Autodesk Inventor part; units mm, degrees
ref_plane "YZ Plane" through (0, 0, 0) normal (1, 0, 0) x (0, 1, 0)
ref_plane "XZ Plane" through (0, 0, 0) normal (0, 1, 0) x (-1, 0, 0)
ref_plane "XY Plane" through (0, 0, 0) normal (0, 0, 1) x (1, 0, 0)
sketch "Sketch1" plane through (0, 0, 0) normal (1, 0, 0) x (0, 1, 0)
  line L0 (-6, -12.5) -> (-6, -12.9)
  arc A0 (-6, -12.9) -> (-5.6, -13.3) centre (-5.6, -12.9) ccw
  line L1 (-5.6, -13.3) -> (-4.9, -13.3)
  arc A1 (-4.9, -13.3) -> (-4.7, -13.1) centre (-4.9, -13.1) ccw
  line L2 (-4.7, -13.1) -> (-4.7, -12.85)
  arc A2 (-4.5, -12.65) -> (-4.7, -12.85) centre (-4.5, -12.85) ccw
  line L3 (-4.5, -12.65) -> (-1.8, -12.65)
  arc A3 (-1.4, -13.05) -> (-1.8, -12.65) centre (-1.8, -13.05) ccw
  line L4 (-1.4, -13.05) -> (-1.4, -18.75)
  line L5 (-1.8, -19.15) -> (-4.5, -19.15)
  arc A4 (-1.8, -19.15) -> (-1.4, -18.75) centre (-1.8, -18.75) ccw
  arc A5 (-4.7, -18.95) -> (-4.5, -19.15) centre (-4.5, -18.95) ccw
  line L6 (-4.7, -18.95) -> (-4.7, -18.7)
  arc A6 (-4.7, -18.7) -> (-4.9, -18.5) centre (-4.9, -18.7) ccw
  line L7 (-4.9, -18.5) -> (-5.6, -18.5)
  arc A7 (-5.6, -18.5) -> (-6, -18.9) centre (-5.6, -18.9) ccw
  line L8 (-6, -18.9) -> (-6, -19.5)
  line L9 (-6.5, -6.5) -> (-6.5, -12.5)
  line L10 (-6.5, -12.5) -> (-2.5, -12.5)
  line L11 (-1.05, -19.5) -> (-6.5, -19.5)
  line L12 (-6.5, -19.5) -> (-6.5, -26)
  line L13 (-6.5, -26) -> (-1.05, -26)
  line L14 (-6, -26) -> (-6, -26.6)
  arc A8 (-6, -26.6) -> (-5.6, -27) centre (-5.6, -26.6) ccw
  line L15 (-5.6, -27) -> (-4.9, -27)
  arc A9 (-4.9, -27) -> (-4.7, -26.8) centre (-4.9, -26.8) ccw
  arc A10 (-4.5, -26.35) -> (-4.7, -26.55) centre (-4.5, -26.55) ccw
  line L16 (-4.7, -26.8) -> (-4.7, -26.55)
  line L17 (-4.5, -26.35) -> (-1.8, -26.35)
  arc A11 (-1.4, -26.75) -> (-1.8, -26.35) centre (-1.8, -26.75) ccw
  line L18 (-1.4, -26.75) -> (-1.4, -32.45)
  arc A12 (-1.8, -32.85) -> (-1.4, -32.45) centre (-1.8, -32.45) ccw
  line L19 (-1.8, -32.85) -> (-4.5, -32.85)
  arc A13 (-4.7, -32.65) -> (-4.5, -32.85) centre (-4.5, -32.65) ccw
  line L20 (-4.7, -32.65) -> (-4.7, -32.4)
  arc A14 (-4.7, -32.4) -> (-4.9, -32.2) centre (-4.9, -32.4) ccw
  line L21 (-4.9, -32.2) -> (-5.6, -32.2)
  arc A15 (-5.6, -32.2) -> (-6, -32.6) centre (-5.6, -32.6) ccw
  line L22 (-6, -32.6) -> (-6, -33)
  line L23 (-2.5, -33) -> (-6.5, -33)
  line L24 (-6.5, -33) -> (-6.5, -39)
  line L25 (32.5, 0) -> (0, 0)
  circle A16 centre (0, -6.5) radius 4.75
  circle A17 centre (32.5, -6.5) radius 4.75
  circle A18 centre (0, -39) radius 4.75
  circle A19 centre (32.5, -39) radius 4.75
  line L26 (39, -26) -> (39, -19.5)
  line L27 (39, -12.5) -> (39, -6.5)
  line L28 (39, -39) -> (39, -33)
  line L29 (26.5, -45.5) -> (32.5, -45.5)
  line L30 (0, -45.5) -> (6, -45.5)
  line L31 (13, -45.5) -> (19.5, -45.5)
  circle A20 centre (16.25, -22.75) radius 15
  circle A21 centre (16.2588, 5.0016) radius 2.5
  circle A22 centre (16.25, -50.5) radius 2.5
  circle A23 centre (16.25, -22.75) radius 5
  circle A24 centre (16.25, -22.75) radius 8.45
  line L32 (24.75, -27.6575) -> (24.75, -17.8425)
  line L33 (44, 10) -> (-11.5, 10)
  line L34 (-11.5, 10) -> (-11.5, -55.5)
  line L35 (-11.5, -55.5) -> (44, -55.5)
  line L36 (44, -55.5) -> (44, 10)
  line L37 (-11.5, 30) -> (44, 30)
  line L38 (-11.5, -75.5) -> (-11.5, 30)
  line L39 (44, 30) -> (44, -75.5)
  line L40 (44, -75.5) -> (-11.5, -75.5)
  circle A25 centre (16.25, -65.5) radius 5
  circle A26 centre (16.25, 20) radius 5
  arc A27 (11.25, -55.5) -> (21.25, -55.5) centre (16.25, -55.5) ccw
  line L41 (21.25, 10) -> (21.25, -55.5)
  line L42 (11.25, -55.5) -> (11.25, 10)
  arc A28 (21.25, 10) -> (11.25, 10) centre (16.25, 10) ccw
  line L43 (21.25, -45.5) -> (11.25, -45.5)
  point P0 (21.25, 0)
  point P1 (11.25, 0)
extrude "Extrusion1" add sketch "Sketch1" along normal blind 10 contours L41 A20 L42 L25 | L41 A24 L42 A20 | L41 A23 L42 A24 | L42 A24 L41 A20 | A20 L41 L43 L31 L42 | A23 | L41 A24 L42 A23
extrude "Extrusion2" add sketch "Sketch1" along normal blind 5 contours L25 L42 L33 L41 | L43 L31 L41 L35 L42
sketch "Sketch2" plane through (10, 11.25, 0) normal (0, 0, 1) x (1, 0, 0)
  line L0 (0, 10) -> (0, 0)
  circle A0 centre (0, 5) radius 7.5
  line L1 (0, 5) -> (11.155, 5)
  line L2 (-5, 10) -> (0, 10)
  line L3 (0, 10) -> (7.5, 5)
  line L4 (7.5, 5) -> (0, 0)
  point P0 (-10, -11.25)
  dimension "d4" = 15
extrude "Extrusion3" add sketch "Sketch2" against normal up to surface (45.5 mm away) contours L3 L1 L0 | L1 L4 L0
properties part number "Cuchilla"
Read the model definition and answer for the solid it produces. Units are mm, in the model's axes. A direction names the side the tool comes from. Give positions to 0.01 mm unless a question says otherwise; leave off trailing zeros. Write each loop counter-clockwise with the first axis right and the second up, starting at its lowest first coordinate (ties: lowest second). Pieces come first, ordered by that corner, then holes. Notation, with made-up numbers: (67, 50) - (84, 50) arc R15 cw to (84, 65) - close; hole circle Ø2 at (71.25, -22.75). An arc over 180 degrees is marked (long way). Return JSON: item names as keys, results as strings.
Q1. A cutting plane is placed at C-C, the plane x = 9.25. Determine the outline of the cut face in (y, z).
Reply:
{"outline": "(11.25, -45.5) - (21.25, -45.5) - (21.25, 0) - (11.25, 0) - close"}
Q2. Given P1, Ø1, axis at x = 14.5, y = 19.5, coming from the +Z side; P2, Ø3, axis at x = 9, y = 14, coming from the +Z side; P3, Ø5, axis at y = 18, z = 3, coming from the +X side; P4, Ø1.5, axis at x = 11.5, z = -17.5, coming from the +Y side, each flat-ended and moving along its own axis, determine where each tip first touches the part or whether it passes through.
Reply:
{"P1": "through", "P2": "z = 0", "P3": "x = 5", "P4": "y = 20.75"}
Q3. For a pull along Y with two mould halves and no side action, classify faces 4 (the face through (13.802, 13.785, -22.432)), 5 (the face through (10, 16, 0)), 6 (the face through (2.465, 13.752, -50.61)), 7 (the face through (2.465, 18.568, 5.959)) as released by +Y, released by -Y, zero draft, split by the parting line, or undercut.
Reply:
{"face 4": "released by -Y", "face 5": "zero draft", "face 6": "undercut", "face 7": "undercut"}
Q4. For faces 1 (the face through (5, 15, -48)), 2 (the face through (5, 14, 7)), 3 (the face through (2, 16, 10)), determine the directions among +Z, -Z, +X, -X, +Y, -Y from which every point of the face is accessible in a straight line to the end or side of a thin tool.
Reply:
{"face 1": "-Z, +X, +Y, -Y", "face 2": "+Z, +X, +Y, -Y", "face 3": "+Z, +X, -X, +Y, -Y"}
Q5. A cutting plane is placed at B-B, the plane z = -25.5. Determine the outline of the cut face in (x, y).
Reply:
{"outline": "(0, 11.25) - (10, 11.25) - (17.5, 16.25) - (10, 21.25) - (0, 21.25) - close"}
Q6. A cutting plane is placed at D-D, the plane z = 1. Determine the outline of the cut face in (x, y).
Reply:
{"outline": "(0, 11.25) - (5, 11.25) - (5, 21.25) - (0, 21.25) - close"}
Q7. A cutting plane is placed at A-A, the plane z = -50.5. Determine the outline of the cut face in (x, y), and give its area (3 significant figures).
Reply:
{"outline": "(0, 11.25) - (5, 11.25) - (5, 13.75) - (0, 13.75) - close; (0, 18.75) - (5, 18.75) - (5, 21.25) - (0, 21.25) - close", "area": "25.0 mm²"}
Q8. Consider line 1 along Z through (x, y) = (4, 16.5); line 2 along Z through (x, y) = (3, 17.25); line 3 along X through (y, z) = (20.25, -47). Determine where each line is inside the solid, lowest interval first. Write a range as [from, to].
Reply:
{"line 1": "[-55.5, -52.99], [-48.01, 2.51], [7.49, 10]", "line 2": "[-55.5, -52.79], [-48.21, 2.71], [7.3, 10]", "line 3": "[0, 5]"}
